Read the model definition and answer for the solid it produces. Units are mm, in the model's axes. A direction names the side the tool comes from. Coordinates: 2 decimals unless noted, no trailing zeros. Order: outer loops, then holes, each group sorted by start corner. A loop starts at its lowest first (then second) coordinate and runs counter-clockwise, first axis right, second up. Notation, with made-up numbers: (0.25, 37) -> (19.25, 37) arc R10 ccw to (19.25, 54) -> close; hole circle Ø7 at (15, 51.25). An arc over 180 degrees is marked (long way). Use CSV: the item, a comma, the result in double quotes.
```python
from build123d import *

# Parameters (mm, degrees)
SZKIC1_W                       = 40
SZKIC1_H                       = 14
SZKIC1_R                       = 2
DODANIE_WYCI_GNI_CIE1_DEPTH    = 10.77
SZKIC2_W                       = 56
SZKIC2_H                       = 14
DODANIE_WYCI_GNI_CIE2_DEPTH    = 20.3
SZKIC5_R                       = 2.25
WYTNIJ_WYCI_GNI_CIE2_DEPTH     = 14
SZKIC8_W                       = 56
SZKIC8_H                       = 10.77
DODANIE_WYCI_GNI_CIE3_DEPTH    = 14
WYTNIJ_WYCI_GNI_CIE3_START     = -14
WYTNIJ_WYCI_GNI_CIE3_OUTLINE_W = 42
WYTNIJ_WYCI_GNI_CIE3_OUTLINE_H = 21
WYTNIJ_WYCI_GNI_CIE3_DEPTH     = 14
SZKIC12_R                      = 2.25
DODANIE_WYCI_GNI_CIE4_DEPTH    = 18
WYTNIJ_WYCI_GNI_CIE1_DEPTH     = 5
SZKIC9_R                       = 2.2
WYTNIJ_WYCI_GNI_CIE4_DEPTH     = 21
SZKIC10_W                      = 56
SZKIC10_H                      = 21
WYTNIJ_WYCI_GNI_CIE5_DEPTH     = 17
SZKIC13_W                      = 21
SZKIC13_H                      = 15
DODANIE_WYCI_GNI_CIE5_DEPTH    = 0.7
SZKIC16_W                      = 21
SZKIC16_H                      = 15
DODANIE_WYCI_GNI_CIE7_DEPTH    = 0.7


# Read off the part's stored shape, not the designer's step: Wytnij-wyciągnięcie3
with BuildPart() as part:
    # Szkic1 → Dodanie-wyciągnięcie1 (new body)
    with BuildSketch(Plane.XY):
        Rectangle(SZKIC1_W, SZKIC1_H)
        with Locations((-14, 0)):
            Circle(SZKIC1_R, mode=Mode.SUBTRACT)
        with Locations((14, 0)):
            Circle(SZKIC1_R, mode=Mode.SUBTRACT)
    extrude(amount=DODANIE_WYCI_GNI_CIE1_DEPTH)

    # Szkic2 → Dodanie-wyciągnięcie2 (add)
    with BuildSketch(Plane.XY.offset(10.77)):
        Rectangle(SZKIC2_W, SZKIC2_H)
    extrude(amount=DODANIE_WYCI_GNI_CIE2_DEPTH)

    # Szkic5 → Wytnij-wyciągnięcie2 (cut)
    with BuildSketch(Plane(origin=(0, 7, 0), x_dir=(1, 0, 0), z_dir=(0, 1, 0))):
        with Locations(Location((-24, -15.92, 0), (0, 0, 180))):
            Circle(SZKIC5_R)
        with Locations(Location((24, -15.92, 0), (0, 0, 180))):
            Circle(SZKIC5_R)
        with Locations(Location((24, -25.92, 0), (0, 0, 180))):
            Circle(SZKIC5_R)
        with Locations(Location((-24, -25.92, 0), (0, 0, 180))):
            Circle(SZKIC5_R)
    extrude(amount=-WYTNIJ_WYCI_GNI_CIE2_DEPTH, mode=Mode.SUBTRACT)

    # Szkic8 → Dodanie-wyciągnięcie3 (add)
    with BuildSketch(Plane(origin=(0, 7, 0), x_dir=(1, 0, 0), z_dir=(0, 1, 0))):
        with Locations((0, -5.385)):
            Rectangle(SZKIC8_W, SZKIC8_H)
    extrude(amount=-DODANIE_WYCI_GNI_CIE3_DEPTH)

    # Wytnij-wyciągnięcie3 outline → Wytnij-wyciągnięcie3 (cut)
    with BuildSketch(Plane(origin=(0, 7, 0), x_dir=(1, 0, 0), z_dir=(0, 1, 0)).offset(WYTNIJ_WYCI_GNI_CIE3_START)):
        with Locations((-0.124911353, -20.57)):
            Rectangle(WYTNIJ_WYCI_GNI_CIE3_OUTLINE_W, WYTNIJ_WYCI_GNI_CIE3_OUTLINE_H)
    extrude(amount=WYTNIJ_WYCI_GNI_CIE3_DEPTH, mode=Mode.SUBTRACT)

    # Szkic12 → Dodanie-wyciągnięcie4 (add)
    with BuildSketch(Plane.XZ.offset(7)):
        Polygon((20.875088647, 31.07), (20.875088647, 10.07), (-21.124911353, 10.07), (-21.124911353, 31.07), (-28, 31.07), (-28, 0), (28, 0), (28, 31.07), align=None)
        with Locations(Location((-24, 25.92, 0), (0, 0, 180))):
            Circle(SZKIC12_R, mode=Mode.SUBTRACT)
        with Locations(Location((24, 25.92, 0), (0, 0, 180))):
            Circle(SZKIC12_R, mode=Mode.SUBTRACT)
        with Locations(Location((-24, 15.92, 0), (0, 0, 180))):
            Circle(SZKIC12_R, mode=Mode.SUBTRACT)
        with Locations(Location((24, 15.92, 0), (0, 0, 180))):
            Circle(SZKIC12_R, mode=Mode.SUBTRACT)
    extrude(amount=DODANIE_WYCI_GNI_CIE4_DEPTH)

    # Szkic4 → Wytnij-wyciągnięcie1 (cut)
    with BuildSketch(Plane.XY.offset(10.07)):
        Polygon((-16.078460969, 3.6), (-18.156921938, 0), (-16.078460969, -3.6), (-11.921539031, -3.6), (-9.843078062, 0), (-11.921539031, 3.6), align=None)
        Polygon((11.921539031, 3.6), (9.843078062, 0), (11.921539031, -3.6), (16.078460969, -3.6), (18.156921938, 0), (16.078460969, 3.6), align=None)
    extrude(amount=-WYTNIJ_WYCI_GNI_CIE1_DEPTH, mode=Mode.SUBTRACT)

    # Szkic9 → Wytnij-wyciągnięcie4 (cut)
    with BuildSketch(Plane.XY.offset(10.07)):
        with Locations((-14, 0)):
            Circle(SZKIC9_R)
        with Locations((14, 0)):
            Circle(SZKIC9_R)
    extrude(amount=-WYTNIJ_WYCI_GNI_CIE4_DEPTH, mode=Mode.SUBTRACT)

    # Szkic10 → Wytnij-wyciągnięcie5 (cut)
    with BuildSketch(Plane(origin=(0, 7, 0), x_dir=(1, 0, 0), z_dir=(0, 1, 0))):
        with Locations((0, -20.57)):
            Rectangle(SZKIC10_W, SZKIC10_H)
    extrude(amount=-WYTNIJ_WYCI_GNI_CIE5_DEPTH, mode=Mode.SUBTRACT)

    # Szkic13 → Dodanie-wyciągnięcie5 (add)
    with BuildSketch(Plane(origin=(-21.124911353, 0, 0), x_dir=(0, 0, -1), z_dir=(1, 0, 0))):
        with Locations((-20.57, -17.5)):
            Rectangle(SZKIC13_W, SZKIC13_H)
    extrude(amount=DODANIE_WYCI_GNI_CIE5_DEPTH)

    # Szkic16 → Dodanie-wyciągnięcie7 (add)
    with BuildSketch(Plane.ZY.offset(-20.875088647)):
        with Locations((20.57, -17.5)):
            Rectangle(SZKIC16_W, SZKIC16_H)
    extrude(amount=DODANIE_WYCI_GNI_CIE7_DEPTH)


solid = part.part
```
Item 1: A tool of negligible diameter and unlimited length cuts with its end or side. For faces 5 (the flat face through (11, 2, 8)), 6 (the flat face through (-20.425, -17, 21)), 7 (the flat face through (24, -10, 20)), from which of +Z, -Z, +X, -X, +Y, -Y can it reach the whole face along a straight path? Write none if from no direction.
Return value:
face 5,"+Z"
face 6,"+Z, +Y, -Y"
face 7,"+Z, +X, -X, +Y"
Item 2: Straight lines are drawn through the part: line 1 along Z through (x, y) = (24, -17.75); line 2 along X through (y, z) = (-20, 23); line 3 along X through (y, z) = (-13, 15.92). For each, find the intervals that lie inside material, in ascending order.
Return value:
line 1,"z = 0 to 13.67, 18.17 to 23.67, 28.17 to 31.07"
line 2,"x = -28 to -20.42, 20.18 to 28"
line 3,"x = -28 to -26.25, -21.75 to -20.42, 20.18 to 21.75, 26.25 to 28"
Item 3: Each of these flat-tipped pins is pushed along its axis until it touches: P1, Ø3.5, axis at x = 24, z = 15.92, coming from the +Y side (1 decimal); P2, Ø8, axis at x = 16, y = 2, coming from the +Z side; P3, Ø2, axis at x = -12.5, y = 0.5, coming from the +Z side; P4, Ø8.5, axis at x = -24, z = 24, coming from the +Y side. Where does it stop, or does it pass through?
Return value:
P1,"passes through"
P2,"stops at z = 10.07"
P3,"stops at z = 5.07"
P4,"stops at y = -10"
Item 4: Find section A-A, the plane x = -14. Give the vertices of the cut face in (y, z), then the cut area to 3 significant figures.
Return value:
outline,"(-25, 0) -> (-2.2, 0) -> (-2.2, 5.07) -> (-3.6, 5.07) -> (-3.6, 10.07) -> (-25, 10.07) -> close; (2.2, 0) -> (7, 0) -> (7, 10.07) -> (3.6, 10.07) -> (3.6, 5.07) -> (2.2, 5.07) -> close"
area,"264 mm^2"
Item 5: Find section B-B, the plane z = 22. Give the vertices of the cut face in (x, y).
Return value:
outline,"(-28, -25) -> (-20.42, -25) -> (-20.42, -10) -> (-28, -10) -> close; (20.18, -25) -> (28, -25) -> (28, -10) -> (20.18, -10) -> close"
Item 6: Find section D-D, the plane x = 24. Give the vertices of the cut face in (y, z).
Return value:
outline,"(-25, 0) -> (7, 0) -> (7, 10.07) -> (-10, 10.07) -> (-10, 13.67) -> (-25, 13.67) -> close; (-25, 18.17) -> (-10, 18.17) -> (-10, 23.67) -> (-25, 23.67) -> close; (-25, 28.17) -> (-10, 28.17) -> (-10, 31.07) -> (-25, 31.07) -> close"
Item 7: Find section C-C, the plane z = 15.92. Give the vertices of the cut face in (x, y).
Return value:
outline,"(-28, -25) -> (-26.25, -25) -> (-26.25, -10) -> (-28, -10) -> close; (-21.75, -25) -> (-20.42, -25) -> (-20.42, -10) -> (-21.75, -10) -> close; (20.18, -25) -> (21.75, -25) -> (21.75, -10) -> (20.18, -10) -> close; (26.25, -25) -> (28, -25) -> (28, -10) -> (26.25, -10) -> close"
Item 8: The mould has two halves that part along X. Classify faces 1 (the flat face through (28, -12, 12)), 2 (the flat face through (17, -2, 8)), 3 (the flat face through (24, -18, 31.07)), 4 (the flat face through (17, 2, 8)): +X half, -X half, draft (parallel to the pull), parting line (faces both ways), or undercut.
Return value:
face 1,"+X half"
face 2,"undercut"
face 3,"draft"
face 4,"undercut"
